Read the model definition and answer for the solid it produces. Units are mm, in the model's axes. Face numbers are marked on the shaded views. A direction names the side the tool comes from. Round coordinates to 2 decimals unless told otherwise and drop trailing zeros. Order: outer loops, then holes, each group sorted by start corner. A loop starts at its lowest first (then second) coordinate and runs counter-clockwise, first axis right, second up. Notation, with made-up numbers: (30, -30) - (69, -30) arc R19 ccw to (69, -1) - close; hole circle Ø3 at (-14.5, 8). An arc over 180 degrees is marked (long way). Answer as a JSON object with one key per item and string values. Group by question number.
Q1. Given pin 1 Ø7.5 at (x, z) = (3.5, -30) entering from -Y; pin 2 Ø5 at (x, z) = (6.35, -44.45) entering from -Y; pin 3 Ø1.5 at (x, z) = (-2, 6) entering from -Y, each flat-ended and moving along its own axis, determine where each tip first touches the part or whether it passes through.
Q2. A tool of negligible diameter and unlimited length cuts with its end or side. For the marked faces 1, 2 and 3, from which of +Z, -Z, +X, -X, +Y, -Y can it reach the whole face along a straight path? Write none if from no direction.
Q3. A cutting plane is placed at A-A on z = -44.45. Determine the outline of the cut face in (x, y), and give its area (3 significant figures).
Q4. Consider line 1 (X direction, y = -2.2, z = -44.45); line 2 (Z direction, x = -6.35, y = -2); line 3 (Z direction, x = 6, y = -6). Determine where each line is inside the solid, lowest interval first.
Q5. A cutting plane is placed at B-B on y = -4.5. Determine the outline of the cut face in (x, z), and give its area (3 significant figures).
Q6. A cutting plane is placed at D-D on z = 7. Determine the outline of the cut face in (x, y).
```python
from build123d import *

# Parameters (mm, degrees)
F0_W           = 25.4
F0_H           = 50.8
F1_DEPTH       = 15.875
F2_R           = 3.048
F3_DEPTH       = 12.7
F4_W           = 7.9375
F4_H           = 34.925
F5_DEPTH       = 25.4
F6_R           = 3.175
F8_D           = 3.6576
F8_CSINK_D     = 7.7978
F8_CSINK_ANGLE = 82
F9_SIZE        = 2.54


with BuildPart() as f1:
    # F0 (on Front) → F1 (new body)
    with BuildSketch(Plane.XZ):
        with Locations((0, -25.4)):
            Rectangle(F0_W, F0_H)
    extrude(amount=F1_DEPTH)

    # F2 (on face) → F3 (join)
    with BuildSketch(Plane.XY):
        with Locations((0, -10.16)):
            Circle(F2_R)
    extrude(amount=F3_DEPTH)

    # F4 (on face) → F5 (cut, through all)
    with BuildSketch(Plane.YZ.offset(12.7)):
        with Locations((-11.90625, -33.3375)):
            Rectangle(F4_W, F4_H)
    extrude(amount=-F5_DEPTH, mode=Mode.SUBTRACT)

    # F6
    f6_edges = [f1.edges().sort_by_distance(p)[0] for p in [
        (12.7, -15.875, -7.9375),
        (-12.7, -15.875, -7.9375),
        (0, -7.9375, -15.875),
    ]]
    fillet(f6_edges, radius=F6_R)

    # F8 (through all)
    with Locations(Plane.XZ.offset(7.9375)):
        with Locations((-6.35, -31.75), (6.35, -31.75), (6.35, -44.45), (-6.35, -44.45)):
            CounterSinkHole(F8_D / 2, F8_CSINK_D / 2, counter_sink_angle=F8_CSINK_ANGLE)

    # F9
    f9_edges = [f1.edges().sort_by_distance(p)[0] for p in [
        (0, -15.875, 0),
    ]]
    chamfer(f9_edges, length=F9_SIZE)


solid = f1.part
```
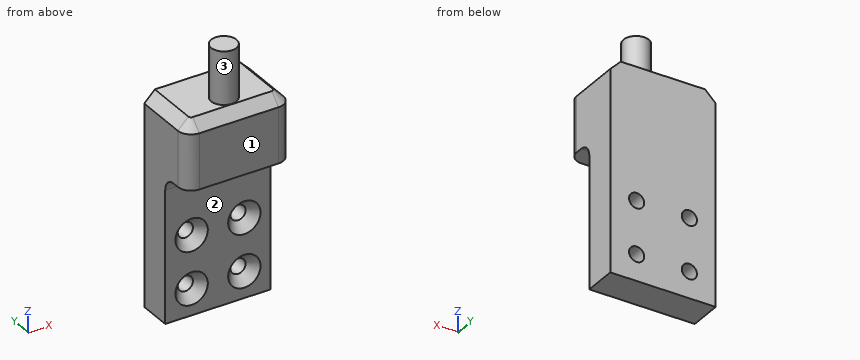
Result set:
{
 "1": {"pin 1": "stops at y = -7.94", "pin 2": "stops at y = -6.33", "pin 3": "stops at y = -12.94"},
 "2": {"face 1": "+Z, -Z, +X, -X, -Y", "face 2": "-Z, +X, -X, -Y", "face 3": "+Z"},
 "3": {"outline": "(-12.7, -7.94) - (-10.25, -7.94) - (-8.18, -5.56) - (-8.18, 0) - (-12.7, 0) - close; (-4.52, -5.56) - (-2.45, -7.94) - (2.45, -7.94) - (4.52, -5.56) - (4.52, 0) - (-4.52, 0) - close; (8.18, -5.56) - (10.25, -7.94) - (12.7, -7.94) - (12.7, 0) - (8.18, 0) - close", "area": "134 mm²"},
 "4": {"line 1": "x = -12.7 to -8.18, -4.52 to 4.52, 8.18 to 12.7", "line 2": "z = -50.8 to -46.28, -42.62 to -33.58, -29.92 to 0", "line 3": "z = -50.8 to -46.64, -42.26 to -33.94, -29.56 to 0"},
 "5": {"outline": "(-12.7, -50.8) - (12.7, -50.8) - (12.7, -2.54) - (10.16, 0) - (-10.16, 0) - (-12.7, -2.54) - close; hole circle Ø3.66 at (-6.35, -44.45); hole circle Ø3.66 at (-6.35, -31.75); hole circle Ø3.66 at (6.35, -44.45); hole circle Ø3.66 at (6.35, -31.75)", "area": "1,240 mm²"},
 "6": {"outline": "circle Ø6.1 at (0, -10.16)"}
}
